Verification items for the finished model (mm, model axes). A direction names the side the tool comes from. Round coordinates to 2 decimals unless told otherwise and drop trailing zeros. Order: outer loops, then holes, each group sorted by start corner. A loop starts at its lowest first (then second) coordinate and runs counter-clockwise, first axis right, second up. Notation, with made-up numbers: (-7.5, 47) -> (29.5, 47) arc R25 cw to (29.5, 67) -> close; hole circle Ø10 at (53.5, 18.5). An arc over 180 degrees is marked (long way). Put each result on its own line as item: value.
from build123d import *

# Parameters (mm, degrees)
SKETCH1_W           = 450
SKETCH1_H           = 350
BOSS_EXTRUDE1_DEPTH = 10
SKETCH2_R           = 3
CUT_EXTRUDE1_DEPTH  = 10
SKETCH3_W           = 10
SKETCH3_H           = 120
CUT_EXTRUDE2_DEPTH  = 10
FILLET1_R           = 3
FILLET2_R           = 3
FILLET3_R           = 10
SKETCH5_R           = 3
BOSS_EXTRUDE3_DEPTH = 10
SKETCH6_R           = 3
BOSS_EXTRUDE4_DEPTH = 10
SKETCH7_R           = 1.5
CUT_EXTRUDE3_DEPTH  = 10


with BuildPart() as part:
    # Sketch1 → Boss-Extrude1 (new body)
    with BuildSketch(Plane(origin=(0, 0, 0), x_dir=(1, 0, 0), z_dir=(0, 1, 0))):
        Rectangle(SKETCH1_W, SKETCH1_H)
    extrude(amount=BOSS_EXTRUDE1_DEPTH)

    # Sketch2 → Cut-Extrude1 (cut)
    with BuildSketch(Plane(origin=(0, 10, 0), x_dir=(1, 0, 0), z_dir=(0, 1, 0))):
        with Locations(Location((-215, -135, 0), (0, 0, 270))):
            Circle(SKETCH2_R)
        with Locations(Location((-205, 0.370879822, 0), (0, 0, 270))):
            Circle(SKETCH2_R)
        with Locations(Location((-215, 135, 0), (0, 0, 270))):
            Circle(SKETCH2_R)
        with Locations(Location((215, 135, 0), (0, 0, 270))):
            Circle(SKETCH2_R)
        with Locations(Location((205, 0, 0), (0, 0, 270))):
            Circle(SKETCH2_R)
        with Locations(Location((215, -135, 0), (0, 0, 270))):
            Circle(SKETCH2_R)
        with Locations(Location((-185, 170, 0), (0, 0, 270))):
            Circle(SKETCH2_R)
        with Locations(Location((0, 170, 0), (0, 0, 270))):
            Circle(SKETCH2_R)
        with Locations(Location((185, 170, 0), (0, 0, 270))):
            Circle(SKETCH2_R)
    extrude(amount=-CUT_EXTRUDE1_DEPTH, mode=Mode.SUBTRACT)

    # Sketch3 → Cut-Extrude2 (cut)
    with BuildSketch(Plane(origin=(0, 10, 0), x_dir=(1, 0, 0), z_dir=(0, 1, 0))):
        with Locations((-220, -5)):
            Rectangle(SKETCH3_W, SKETCH3_H)
        with Locations((220, -5)):
            Rectangle(SKETCH3_W, SKETCH3_H)
    extrude(amount=-CUT_EXTRUDE2_DEPTH, mode=Mode.SUBTRACT)

    # Fillet1
    fillet1_edges = [part.edges().sort_by_distance(p)[0] for p in [
        (-215, 5, -55),
        (-215, 5, 65),
        (215, 5, 65),
        (215, 5, -55),
    ]]
    fillet(fillet1_edges, radius=FILLET1_R)

    # Fillet2
    fillet2_edges = [part.edges().sort_by_distance(p)[0] for p in [
        (-225, 5, 65),
        (-225, 5, -55),
        (225, 5, -55),
        (225, 5, 65),
    ]]
    fillet(fillet2_edges, radius=FILLET2_R)

    # Fillet3
    fillet3_edges = [part.edges().sort_by_distance(p)[0] for p in [
        (-225, 5, -175),
        (225, 5, -175),
        (225, 5, 175),
        (-225, 5, 175),
    ]]
    fillet(fillet3_edges, radius=FILLET3_R)

    # Sketch5 → Boss-Extrude3 (add)
    with BuildSketch(Plane(origin=(0, 10, 0), x_dir=(1, 0, 0), z_dir=(0, 1, 0))):
        with Locations((-215, 135)):
            Circle(SKETCH5_R)
    extrude(amount=-BOSS_EXTRUDE3_DEPTH)

    # Sketch6 → Boss-Extrude4 (add)
    with BuildSketch(Plane(origin=(0, 10, 0), x_dir=(1, 0, 0), z_dir=(0, 1, 0))):
        with Locations((-185, 170)):
            Circle(SKETCH6_R)
        with Locations((0, 170)):
            Circle(SKETCH6_R)
        with Locations((185, 170)):
            Circle(SKETCH6_R)
        with Locations((215, 135)):
            Circle(SKETCH6_R)
        with Locations((205, 0)):
            Circle(SKETCH6_R)
        with Locations((215, -135)):
            Circle(SKETCH6_R)
        with Locations((-215, -135)):
            Circle(SKETCH6_R)
        with Locations((-205, 0.370879822)):
            Circle(SKETCH6_R)
    extrude(amount=-BOSS_EXTRUDE4_DEPTH)

    # Sketch7 → Cut-Extrude3 (cut)
    with BuildSketch(Plane(origin=(0, 10, 0), x_dir=(1, 0, 0), z_dir=(0, 1, 0))):
        with Locations(Location((-185, 170, 0), (0, 0, 270))):
            Circle(SKETCH7_R)
        with Locations(Location((-215.140831726, 135, 0), (0, 0, 270))):
            Circle(SKETCH7_R)
        with Locations(Location((-205, 0.381414612, 0), (0, 0, 270))):
            Circle(SKETCH7_R)
        with Locations(Location((-215, -135, 0), (0, 0, 270))):
            Circle(SKETCH7_R)
        with Locations(Location((215, -135, 0), (0, 0, 270))):
            Circle(SKETCH7_R)
        with Locations(Location((205, 0.370879822, 0), (0, 0, 270))):
            Circle(SKETCH7_R)
        with Locations(Location((215, 135, 0), (0, 0, 270))):
            Circle(SKETCH7_R)
        with Locations(Location((0, 170, 0), (0, 0, 270))):
            Circle(SKETCH7_R)
        with Locations(Location((185, 170, 0), (0, 0, 270))):
            Circle(SKETCH7_R)
    extrude(amount=-CUT_EXTRUDE3_DEPTH, mode=Mode.SUBTRACT)


solid = part.part
Item 1: Tool access check on faces 4 (the flat face through (-215, 5, 6)), 5 (the flat face through (-3, 0, -2)). Record the directions out of +Z, -Z, +X, -X, +Y, -Y that give a thin tool (end or side, any length) a straight path to the whole face; none if there is none.
Check sheet entries:
face 4: -X, +Y, -Y
face 5: +Z, -Z, +X, -X, -Y
Item 2: Section check A-A on y = 8. State how many separate pieces and enclosed holes the cut face has, then the cut area to 3 significant figures.
Check sheet entries:
separate pieces: 1
enclosed holes: 9
area: 155,000 mm^2
Item 3: Material ranges on L1, parallel to X at y = 5.75, z = 135; L2, parallel to X at y = 4.25, z = -135; L3, parallel to Z at x = 185, y = 7.75, recorded low to high. Write a range as [from, to].
Check sheet entries:
L1: x = [-225, -216.5], [-213.5, 213.5], [216.5, 225]
L2: x = [-225, -216.64], [-213.64, 213.5], [216.5, 225]
L3: z = [-175, -171.5], [-168.5, 175]
Item 4: Section check B-B on z = 11.5. Record the boundary of the cut face in (x, y), then the cut area to 3 significant figures.
Check sheet entries:
outline: (-215, 0) -> (215, 0) -> (215, 10) -> (-215, 10) -> close
area: 4,300 mm^2
Item 5: Gauge pin test, flat ends, axial feed: pin 1 Ø2 at (x, z) = (22.5, 79) entering from -Y; pin 2 Ø1.8 at (x, z) = (0, -170) entering from +Y (3 decimals); pin 3 Ø5 at (y, z) = (4, -20) entering from -X; pin 4 Ø2 at (x, y) = (-219.5, 3) entering from -Z. Record the tip position at first contact, or that the pin passes through.
Check sheet entries:
pin 1: stops at y = 0
pin 2: passes through
pin 3: stops at x = -215
pin 4: stops at z = -174.37
Item 6: Release check for a two-part mould opening along Z. For faces 1 (the flat face through (215, 5, 6)), 2 (the cylindrical face through (-222.15, 5.07, 171.99)), 3 (the flat face through (-3, 10, -2)) record: +Z half, -Z half, draft (parallel to the pull), parting line (faces both ways), or undercut.
Check sheet entries:
face 1: undercut
face 2: +Z half
face 3: draft
